from build123d import *

# Parameters (mm, degrees)
CROQUIS1_R                 = 13
CROQUIS1_R_2               = 11.05
SALIENTE_EXTRUIR1_DEPTH    = 1
BARRER_L_MINA1_PROFILE_R   = 13.05
BARRER_L_MINA1_PROFILE_R_2 = 11.05


with BuildPart() as part:
    # Croquis1 → Saliente-Extruir1 (new body)
    with BuildSketch(Plane(origin=(0, 0, 0), x_dir=(1, 0, 0), z_dir=(0, 1, 0))):
        with Locations(Location((0, 0, 0), (0, 0, 270))):
            Circle(CROQUIS1_R)
        with Locations(Location((0, 0, 0), (0, 0, 270))):
            Circle(CROQUIS1_R_2, mode=Mode.SUBTRACT)
    extrude(amount=-SALIENTE_EXTRUIR1_DEPTH)

    # Barrer-L_mina1: sweep along a path in Croquis2
    with BuildLine(Plane.XY) as barrer_l_mina1_path:
        Line((0, -1), (0, -21))
        ThreePointArc((0, -21), (2.727754239, -29.625078781), (9.918931196, -35.113211534))
        Line((9.918931196, -35.113211534), (29.677427344, -42.226707859))
    # Barrer-L_mina1 profile (on start of the path) → Barrer-L_mina1 (sweep)
    with BuildSketch(Plane(origin=(0, -1, 0), x_dir=(-1, 0, 0), z_dir=(0, -1, 0))):
        Circle(BARRER_L_MINA1_PROFILE_R)
        Circle(BARRER_L_MINA1_PROFILE_R_2, mode=Mode.SUBTRACT)
    sweep(path=barrer_l_mina1_path.line)


solid = part.part
The listing builds one solid part. Answer for the finished solid, in the listing's coordinates (mm). A direction names the side the tool comes from. Round coordinates to 2 decimals unless told otherwise and drop trailing zeros. Loops run counter-clockwise (first coordinate to the right, second up) from the corner with the lowest first, then second, coordinate; pieces in that order, holes last. Notation, with made-up numbers: M 46,-20.5 L 70,-20.5 A19 cw 70,-7.5 Z; hole C 53,-21 d8. An arc over 180 degrees is marked long. Write each question's results on one line, items separated by ' | '. Start each with the question number.
1) Find section B-B on z = 0. Write down the section's boundary in (x, y), plus the area to 3 significant figures.
2) Find section A-A on z = -10. Write down the section's boundary in (x, y), plus the area to 3 significant figures.
3) Determine the mould class of faces 3 (the cylindrical face through (9.62, -11.14, -8.82)), 4 (the flat face through (26.38, -51.38, 5.86)), 5 (the cylindrical face through (16.479, -48.324, 4.232)) for opening direction Z: pulls with the +Z half, pulls with the -Z half, needs draft (parallel to the pull), parting line crosses it, or undercut.
4) Each of these flat-tipped pins is pushed along its axis until it touches: pin 1 (5 mm diameter, centred on y = -36.5, z = 7, fed in from -X); pin 2 (12 mm diameter, centred on x = 20.5, z = 3, fed in from +Y); pin 3 (1 mm diameter, centred on x = 5, z = -4, fed in from +Y); pin 4 (3 mm diameter, centred on x = 0, y = -47, fed in from -Z). Where does it stop, or does it pass through?
5) Straight lines are drawn through the part: probe 1 along Z at (x, y) = (0, -16); probe 2 along X at (y, z) = (-0.8, 0); probe 3 along Y at (x, z) = (12.5, 5.25). For each, find the intervals that lie inside material, in ascending order.
6) Which of the six approach directions +Z, -Z, +X, -X, +Y, -Y give full straight-line access (tool end or side, diameter ignored) to faces 1 (the cylindrical face through (-7.91, -0.493, -10.316)), 2 (the flat face through (-10, 0, -6))?
Final values:
1) outline: M -13.05,-21 A28.05 ccw 5.5,-47.39 L 25.26,-54.51 L 25.93,-52.62 L 6.18,-45.51 A26.05 cw -11.05,-21 L -11.05,0 L -13,0 L -13,-1 L -13.05,-1 Z; M 11.05,-21 A3.95 ccw 13.66,-24.72 L 33.42,-31.83 L 34.1,-29.95 L 14.34,-22.83 A1.95 cw 13.05,-21 L 13.05,-1 L 13,-1 L 13,0 L 11.05,0 Z | area: 241 mm²
2) outline: M -8.38,-21 A23.38 ccw 7.08,-43 L 26.84,-50.12 L 28.08,-46.65 L 8.33,-39.54 A19.7 cw -4.7,-21 L -4.7,0 L -8.31,0 L -8.31,-1 L -8.38,-1 Z; M 4.7,-21 A10.3 ccw 11.51,-30.69 L 31.27,-37.8 L 32.52,-34.34 L 12.76,-27.22 A6.62 cw 8.38,-21 L 8.38,-1 L 8.31,-1 L 8.31,0 L 4.7,0 Z | area: 445 mm²
3) face 3: parting line crosses it | face 4: needs draft | face 5: undercut
4) pin 1: x = -8.2 | pin 2: y = -23.05 | pin 3: y = -43.93 | pin 4: through
5) probe 1: -13.05 to -11.05, 11.05 to 13.05 | probe 2: -13 to -11.05, 11.05 to 13 | probe 3: -48.74 to -46.38, -25.65 to -22.75
6) face 1: +Y | face 2: +Z, -Z, +X, -X, +Y
